```python
from build123d import *

# Parameters (mm, degrees)
F0_W      = 89
F0_H      = 60
F1_DEPTH  = 2
F2_R      = 3
F2_R_2    = 1.5
F3_DEPTH  = 17
F4_W      = 52
F4_H      = 49
F5_DEPTH  = 2
F6_W      = 4.5
F6_H      = 15
F7_DEPTH  = 2
F8_W      = 14.81
F8_H      = 10
F9_DEPTH  = 2
F11_W     = 17.5
F11_H     = 1.5
F11_W_2   = 8
F12_DEPTH = 10
F11_W_3   = 9.5
F13_DEPTH = 13.5
F14_W     = 1.5
F14_H     = 4
F15_DEPTH = 4
F16_SIZE  = 3.99999
F17_W     = 20
F17_H     = 15
F18_DEPTH = 2
F19_W     = 15
F19_H     = 13
F19_W_2   = 30.315
F19_H_2   = 5.5
F19_W_3   = 13
F19_H_3   = 9
F20_DEPTH = 2
F22_W     = 4.75
F22_H     = 6.5
F22_W_2   = 1
F22_H_2   = 19
F22_H_3   = 17.5
F23_DEPTH = 2
F25_DEPTH = 2
F21_R     = 1.05
F26_DEPTH = 2


# Not quite as in the source:
# - a fillet or chamfer is up to 0.001 mm smaller than in the source, because OpenCascade refuses the exact size
# - a feature of the source that left no trace in its solid (it failed there, or was rolled back) is left out


with BuildPart() as f1:
    # F0 (on Top) → F1 (new body)
    with BuildSketch(Plane.XY):
        Polygon((89, 0), (0, 0), (0, 60), (-5, 60), (-5, 0), (-5, -10), (89, -10), (99, -10), (99, 60), (89, 60), align=None)
        Polygon((-5, 60), (0, 60), (89, 60), (99, 60), (99, 61.5), (-5, 61.5), align=None)
        with Locations((44.5, 30)):
            Rectangle(F0_W, F0_H)
    extrude(amount=F1_DEPTH)

    # F2 (on face) → F3 (join)
    with BuildSketch(Plane(origin=(0, 0, 0), x_dir=(1, 0, 0), z_dir=(0, 0, -1))):
        with Locations((5.5, -5.5)):
            Circle(F2_R)
        with Locations((5.5, -5.5)):
            Circle(F2_R_2, mode=Mode.SUBTRACT)
        with Locations((63.5, -5.5)):
            Circle(F2_R)
        with Locations((63.5, -5.5)):
            Circle(F2_R_2, mode=Mode.SUBTRACT)
        with Locations((5.5, -54.5)):
            Circle(F2_R)
        with Locations((5.5, -54.5)):
            Circle(F2_R_2, mode=Mode.SUBTRACT)
        with Locations((63.5, -54.5)):
            Circle(F2_R)
        with Locations((63.5, -54.5)):
            Circle(F2_R_2, mode=Mode.SUBTRACT)
    extrude(amount=F3_DEPTH)

    # F4 (on face) → F5 (cut, through all)
    with BuildSketch(Plane.XY.offset(2)):
        with Locations((34.5, 34)):
            Rectangle(F4_W, F4_H)
    extrude(amount=-F5_DEPTH, mode=Mode.SUBTRACT)

    # F6 (on face) → F7 (cut, through all)
    with BuildSketch(Plane.XY.offset(2)):
        with Locations((6.25, 30)):
            Rectangle(F6_W, F6_H)
        Polygon((8.5, 9.5), (8.5, 22.5), (4, 22.5), (1.5, 22.5), (1.5, 9.5), align=None)
    extrude(amount=-F7_DEPTH, mode=Mode.SUBTRACT)

    # F8 (on face) → F9 (cut, through all)
    with BuildSketch(Plane.XY.offset(2)):
        with Locations((55.28, -5)):
            Rectangle(F8_W, F8_H)
    extrude(amount=-F9_DEPTH, mode=Mode.SUBTRACT)

    # F11 (on face) → F12 (join)
    with BuildSketch(Plane(origin=(0, 0, 0), x_dir=(1, 0, 0), z_dir=(0, 0, -1))):
        with Locations((34, -0.75)):
            Rectangle(F11_W, F11_H)
        with Locations((55.5, -0.75)):
            Rectangle(F11_W_2, F11_H)
    extrude(amount=F12_DEPTH)

    # F11 (on face) → F13 (join)
    with BuildSketch(Plane(origin=(0, 0, 0), x_dir=(1, 0, 0), z_dir=(0, 0, -1))):
        with Locations((12.5, -0.75)):
            Rectangle(F11_W_3, F11_H)
    extrude(amount=F13_DEPTH)

    # F14 (on face) → F15 (join)
    with BuildSketch(Plane(origin=(0, 0, 0), x_dir=(1, 0, 0), z_dir=(0, 0, -1))):
        with Locations((34, -3.5)):
            Rectangle(F14_W, F14_H)
        with Locations((55.5, -3.5)):
            Rectangle(F14_W, F14_H)
        with Locations((12.5, -3.5)):
            Rectangle(F14_W, F14_H)
    extrude(amount=F15_DEPTH)

    # F16 (size 4 in the source; OpenCascade refuses exactly that, so slightly less here)
    f16_edges = [f1.edges().sort_by_distance(p)[0] for p in [
        (12.5, 5.5, -4),
        (34, 5.5, -4),
        (55.5, 5.5, -4),
    ]]
    chamfer(f16_edges, length=F16_SIZE)

    # F17 (on face) → F18 (cut, through all)
    with BuildSketch(Plane(origin=(0, 0, 0), x_dir=(1, 0, 0), z_dir=(0, 0, -1))):
        with Locations((70.5, -37)):
            Rectangle(F17_W, F17_H)
    extrude(amount=-F18_DEPTH, mode=Mode.SUBTRACT)

    # F19 (on face) → F20 (cut, through all)
    with BuildSketch(Plane(origin=(0, 0, 0), x_dir=(1, 0, 0), z_dir=(0, 0, -1))):
        with Locations((73, -16)):
            Rectangle(F19_W, F19_H)
        with Locations((80.8425, 4.25)):
            Rectangle(F19_W_2, F19_H_2)
        with Locations((74, -52)):
            Rectangle(F19_W_3, F19_H_3)
    extrude(amount=-F20_DEPTH, mode=Mode.SUBTRACT)

    # F22 (on face) → F23 (cut, through all)
    with BuildSketch(Plane.XY):
        with Locations((0.375, -4.25)):
            Rectangle(F22_W, F22_H)
        with Locations((-1.5, 10.5)):
            Rectangle(F22_W_2, F22_H_2)
        with Locations((-1.5, 48.75)):
            Rectangle(F22_W_2, F22_H_3)
    extrude(amount=F23_DEPTH, mode=Mode.SUBTRACT)

    # F24 (on face) → F25 (cut, through all)
    with BuildSketch(Plane.XY.offset(2)):
        Polygon((-3.5, -8.5), (-3.5, 60), (97.5, 60), (97.5, -8.5), (62.685, -8.5), (62.685, -10), (99, -10), (99, 61.5), (-5, 61.5), (-5, -10), (47.875, -10), (47.875, -8.5), align=None)
    extrude(amount=-F25_DEPTH, mode=Mode.SUBTRACT)

    # F21 (on face) → F26 (cut, through all)
    with BuildSketch(Plane.XY.offset(2)):
        with BuildLine():
            ThreePointArc((64, 24.7), (64.7424621202, 25.0075378798), (65.05, 25.75))
            ThreePointArc((65.05, 25.75), (64.7424621202, 26.4924621202), (64, 26.8))
            Line((64, 26.8), (64, 25.75))
            Line((64, 25.75), (64, 24.7))
        make_face()
        with BuildLine():
            Line((64, 25.75), (64, 26.8))
            ThreePointArc((64, 26.8), (62.95, 25.75), (64, 24.7))
            Line((64, 24.7), (64, 25.75))
        make_face()
        with Locations((44, 14.5)):
            Circle(F21_R)
    extrude(amount=-F26_DEPTH, mode=Mode.SUBTRACT)


solid = f1.part
```
Here's how the part is built. I have some questions about the finished solid (model axes, mm). A direction names the side the tool comes from. Give positions to 0.01 mm unless a question says otherwise; leave off trailing zeros. Order: outer loops, then holes, each group sorted by start corner. A loop starts at its lowest first (then second) coordinate and runs counter-clockwise, first axis right, second up. Notation, with made-up numbers: (83.25, 6) - (112.25, 6) arc R14 ccw to (112.25, 29) - close; hole circle Ø8 at (-18.5, -2.75). An arc over 180 degrees is marked (long way). Answer as a JSON object with one key per item and string values. Group by question number.
Item 1: If we mould it in two halves opening along X, with no side actions, what happens to faces 5 (the flat face through (8.5, 48, 1)), 6 (the cylindrical face through (64.93, 5.05, -8.38)), 7 (the flat face through (65, 7, -17)), 8 (the flat face through (97.5, 26, 1))? For each: pulls with the +X half, pulls with the -X half, needs draft (parallel to the pull), parting line crosses it, or undercut.
Item 2: If we section it at A-A on z = -11.5: Give the number of separate pieces and of enclosed holes in the cut face, and give its area (3 significant figures).
Item 3: For P1, Ø8, axis at x = 79, y = 22, coming from the -Z side; P2, Ø6, axis at x = 76, z = -1, coming from the -Y side; P3, Ø10, axis at y = 8, z = -12, coming from the -X side; P4, Ø3, axis at x = 36.5, z = -4, coming from the -Y side, each with a flat end and sliding along its axis, tell me the tip position at first contact or that it passes through.
Item 4: Please list where these lines run through material, in increasing order: probe 1 along X at (y, z) = (54.5, -9.25); probe 2 along Y at (x, z) = (63.5, -8.5); probe 3 along Z at (x, y) = (76, 7.5).
Item 5: If we section it at C-C on y = 11.5: Please give me the cut outline in (x, z), and give its area (3 significant figures).
Item 6: If we section it at D-D on x = 77: Please give me the cut outline in (y, z), and give its area (3 significant figures).
Item 7: Which directions (+Z, -Z, +X, -X, +Y, -Y) give clear straight access to the entire face, cutting with the end or side of a thin tool? Please do faces 1 (the flat face through (65, 56, -17)), 2 (the flat face through (33.25, 3, -2)), 3 (the flat face through (-1, 10, 1)), 4 (the cylindrical face through (5.109, 51.526, -8.381)).
Item 8: If we section it at B-B on x = 31: Please give me the cut outline in (y, z).
Result set:
{
 "1": {"face 5": "undercut", "face 6": "undercut", "face 7": "needs draft", "face 8": "pulls with the +X half"},
 "2": {"separate pieces": "5", "enclosed holes": "4", "area": "99.1 mm²"},
 "3": {"P1": "z = 0", "P2": "y = -8.5", "P3": "x = 2.5", "P4": "y = 0"},
 "4": {"probe 1": "2.5 to 4, 7 to 8.5, 60.5 to 62, 65 to 66.5", "probe 2": "2.5 to 4, 7 to 8.5, 51.5 to 53, 56 to 57.5", "probe 3": "0 to 2"},
 "5": {"outline": "(-3.5, 0) - (-2, 0) - (-2, 2) - (-3.5, 2) - close; (-1, 0) - (1.5, 0) - (1.5, 2) - (-1, 2) - close; (60.5, 0) - (65.5, 0) - (65.5, 2) - (60.5, 2) - close; (80.5, 0) - (97.5, 0) - (97.5, 2) - (80.5, 2) - close", "area": "52.0 mm²"},
 "6": {"outline": "(-8.5, 0) - (-7, 0) - (-7, 2) - (-8.5, 2) - close; (-1.5, 0) - (9.5, 0) - (9.5, 2) - (-1.5, 2) - close; (22.5, 0) - (29.5, 0) - (29.5, 2) - (22.5, 2) - close; (44.5, 0) - (47.5, 0) - (47.5, 2) - (44.5, 2) - close; (56.5, 0) - (60, 0) - (60, 2) - (56.5, 2) - close", "area": "52.0 mm²"},
 "7": {"face 1": "-Z, +X, -X, +Y, -Y", "face 2": "-Z, +Y", "face 3": "+Z, -Z", "face 4": "-Z"},
 "8": {"outline": "(-8.5, 0) - (0, 0) - (0, -10) - (1.5, -10) - (1.5, 0) - (9.5, 0) - (9.5, 2) - (-8.5, 2) - close; (58.5, 0) - (60, 0) - (60, 2) - (58.5, 2) - close"}
}
